from build123d import *

# Parameters (mm, degrees)
SKETCH1_R           = 4.5
BOSS_EXTRUDE1_DEPTH = 6
SKETCH3_R           = 1.6
SKETCH3_R_2         = 0.7
BOSS_EXTRUDE2_DEPTH = 1.6
SKETCH4_R           = 0.8
BOSS_EXTRUDE3_DEPTH = 0.8
BOSS_EXTRUDE4_START = -4
SKETCH5_R           = 0.6
BOSS_EXTRUDE4_DEPTH = 3
CUT_EXTRUDE1_START  = -2
CUT_EXTRUDE1_DEPTH  = 1
CUT_EXTRUDE2_START  = -4
CUT_EXTRUDE2_DEPTH  = 1
FILLET1_R           = 0.3
SKETCH6_R           = 3.2
SKETCH6_R_2         = 2.2
CUT_EXTRUDE4_DEPTH  = 2
SKETCH6_4_R         = 2.2
CUT_EXTRUDE5_DEPTH  = 19.08212732


with BuildPart() as part:
    # Sketch1 → Boss-Extrude1 (new body)
    with BuildSketch(Plane(origin=(0, 0, 0), x_dir=(1, 0, 0), z_dir=(0, 1, 0))):
        with Locations(Location((0, 0, 0), (0, 0, 270))):
            Circle(SKETCH1_R)
    extrude(amount=BOSS_EXTRUDE1_DEPTH)

    # Sketch3 → Boss-Extrude2 (add)
    # profile 1 of 4: a face of its own
    with BuildSketch(Plane.XZ):
        with Locations((-3.25, 5.629165125)):
            Circle(SKETCH3_R)
        with Locations(Location((-3.25, 5.629165125, 0), (0, 0, 270))):
            Circle(SKETCH3_R_2, mode=Mode.SUBTRACT)
    # profile 2 of 4: a face of its own
    with BuildSketch(Plane.XZ):
        with BuildLine():
            ThreePointArc((-1.65, 5.629165125), (-2.835889528, 4.083683803), (-4.635640646, 4.829165125))
            Line((-4.635640646, 4.829165125), (-3.488614731, 2.842457961))
            ThreePointArc((-3.488614731, 2.842457961), (-2.25, 3.897114317), (-0.717333438, 4.442457961))
            Line((-0.717333438, 4.442457961), (-1.864359354, 6.429165125))
            ThreePointArc((-1.864359354, 6.429165125), (-1.704518678, 6.043275597), (-1.65, 5.629165125))
        make_face()
    # profile 3 of 4: a face of its own
    with BuildSketch(Plane.XZ):
        with Locations((-3.25, -5.629165125)):
            Circle(SKETCH3_R)
        with Locations(Location((-3.25, -5.629165125, 0), (0, 0, 270))):
            Circle(SKETCH3_R_2, mode=Mode.SUBTRACT)
    # profile 4 of 4: a face of its own
    with BuildSketch(Plane.XZ):
        with BuildLine():
            ThreePointArc((-0.717333438, -4.442457961), (-2.25, -3.897114317), (-3.488614731, -2.842457961))
            Line((-3.488614731, -2.842457961), (-4.635640646, -4.829165125))
            ThreePointArc((-4.635640646, -4.829165125), (-2.835889528, -4.083683803), (-1.65, -5.629165125))
            ThreePointArc((-1.65, -5.629165125), (-1.704518678, -6.043275597), (-1.864359354, -6.429165125))
            Line((-1.864359354, -6.429165125), (-0.717333438, -4.442457961))
        make_face()
    extrude(amount=-BOSS_EXTRUDE2_DEPTH)

    # Sketch4 → Boss-Extrude3 (add, symmetric)
    with BuildSketch(Plane.XY):
        with BuildLine():
            Line((-3.5, 6), (-6.5, 6))
            ThreePointArc((-6.5, 6), (-7.9, 4.6), (-6.5, 3.2))
            Line((-6.5, 3.2), (-3.5, 3.2))
            Line((-3.5, 3.2), (-3.5, 6))
        make_face()
        with Locations((-6.5, 4.6)):
            Circle(SKETCH4_R, mode=Mode.SUBTRACT)
    extrude(amount=BOSS_EXTRUDE3_DEPTH, both=True)

    # Sketch5 → Boss-Extrude4 (add)
    # profile 1 of 2: a face of its own
    with BuildSketch(Plane(origin=(0, 6, 0), x_dir=(1, 0, 0), z_dir=(0, 1, 0)).offset(BOSS_EXTRUDE4_START)):
        with BuildLine():
            Line((4.108268481, 3.656792323), (1.029929577, 4.380553055))
            ThreePointArc((1.029929577, 4.380553055), (4.5, 0), (1.029929577, -4.380553055))
            Line((1.029929577, -4.380553055), (14.486091549, -1.216820293))
            ThreePointArc((14.486091549, -1.216820293), (15.45, 0), (14.486091549, 1.216820293))
            Line((14.486091549, 1.216820293), (12.664921694, 1.645002916))
            ThreePointArc((12.664921694, 1.645002916), (12.319323987, 1.235134702), (12.080503997, 0.75514018))
            ThreePointArc((12.080503997, 0.75514018), (11.95, 0), (12.080503997, -0.75514018))
            Line((12.080503997, -0.75514018), (4.931081365, -2.436069903))
            ThreePointArc((4.931081365, -2.436069903), (5.5, 0), (4.931081365, 2.436069903))
            ThreePointArc((4.931081365, 2.436069903), (4.560701943, 3.074084869), (4.108268481, 3.656792323))
        make_face()
        with Locations(Location((14.2, 0, 0), (0, 0, 270))):
            Circle(SKETCH5_R, mode=Mode.SUBTRACT)
    # profile 2 of 2: a face of its own
    with BuildSketch(Plane(origin=(0, 6, 0), x_dir=(1, 0, 0), z_dir=(0, 1, 0)).offset(BOSS_EXTRUDE4_START)):
        with BuildLine():
            Line((12.664921694, 1.645002916), (4.108268481, 3.656792323))
            ThreePointArc((4.108268481, 3.656792323), (4.560701943, 3.074084869), (4.931081365, 2.436069903))
            Line((4.931081365, 2.436069903), (12.080503997, 0.75514018))
            ThreePointArc((12.080503997, 0.75514018), (12.319323987, 1.235134702), (12.664921694, 1.645002916))
        make_face()
    extrude(amount=BOSS_EXTRUDE4_DEPTH)

    # Sketch5_3 → Cut-Extrude1 (cut)
    with BuildSketch(Plane(origin=(0, 6, 0), x_dir=(1, 0, 0), z_dir=(0, 1, 0)).offset(CUT_EXTRUDE1_START)):
        with BuildLine():
            Line((12.664921694, 1.645002916), (4.108268481, 3.656792323))
            ThreePointArc((4.108268481, 3.656792323), (4.560701943, 3.074084869), (4.931081365, 2.436069903))
            Line((4.931081365, 2.436069903), (12.080503997, 0.75514018))
            ThreePointArc((12.080503997, 0.75514018), (12.319323987, 1.235134702), (12.664921694, 1.645002916))
        make_face()
    extrude(amount=CUT_EXTRUDE1_DEPTH, mode=Mode.SUBTRACT)

    # Sketch5_4 → Cut-Extrude2 (cut)
    with BuildSketch(Plane(origin=(0, 6, 0), x_dir=(1, 0, 0), z_dir=(0, 1, 0)).offset(CUT_EXTRUDE2_START)):
        with BuildLine():
            Line((12.664921694, 1.645002916), (4.108268481, 3.656792323))
            ThreePointArc((4.108268481, 3.656792323), (4.560701943, 3.074084869), (4.931081365, 2.436069903))
            Line((4.931081365, 2.436069903), (12.080503997, 0.75514018))
            ThreePointArc((12.080503997, 0.75514018), (12.319323987, 1.235134702), (12.664921694, 1.645002916))
        make_face()
    extrude(amount=CUT_EXTRUDE2_DEPTH, mode=Mode.SUBTRACT)

    # Fillet1
    fillet1_edges = [part.edges().sort_by_distance(p)[0] for p in [
        (4.931081365, 3.5, 2.436069903),
        (12.080503997, 3.5, 0.75514018),
        (4.931081365, 3.5, -2.436069903),
        (12.080503997, 3.5, -0.75514018),
    ]]
    fillet(fillet1_edges, radius=FILLET1_R)

    # Sketch6 → Cut-Extrude4 (cut)
    with BuildSketch(Plane(origin=(0, 6, 0), x_dir=(1, 0, 0), z_dir=(0, 1, 0))):
        with Locations(Location((0, 0, 0), (0, 0, 270))):
            Circle(SKETCH6_R)
        with Locations(Location((0, 0, 0), (0, 0, 270))):
            Circle(SKETCH6_R_2, mode=Mode.SUBTRACT)
    extrude(amount=-CUT_EXTRUDE4_DEPTH, mode=Mode.SUBTRACT)

    # Sketch6_4 → Cut-Extrude5 (cut, through all)
    with BuildSketch(Plane(origin=(0, 6, 0), x_dir=(1, 0, 0), z_dir=(0, 1, 0))):
        with Locations(Location((0, 0, 0), (0, 0, 270))):
            Circle(SKETCH6_4_R)
    extrude(amount=-CUT_EXTRUDE5_DEPTH, mode=Mode.SUBTRACT)


solid = part.part
Source: CAD feature listing. Evaluate the final solid. Frame: model axes, mm. A direction names the side the tool comes from. Round coordinates to 2 decimals unless told otherwise and drop trailing zeros. Order: outer loops, then holes, each group sorted by start corner. A loop starts at its lowest first (then second) coordinate and runs counter-clockwise, first axis right, second up. Notation, with made-up numbers: (-10.5, 31.5) - (36.5, 31.5) arc R9 ccw to (36.5, 47.5) - close; hole circle Ø11 at (89.5, 44.25). An arc over 180 degrees is marked (long way). Use a Markdown table: item, result. Add a question column.
1. Section query B-B (z = 5.75). Return the cut outline in (x, y), then the cut area to 3 significant figures.
2. Set-up query: faces 1 (the flat face through (-4.07, 0.79, 3.85)), 2 (the flat face through (8, 4, -2)), 3 (the flat face through (-2, 1.6, -5)), 4 (the flat face through (8, 3, -2)), 5 (the cylindrical face through (-4.39, 2.96, -0.98)). Return all of +Z, -Z, +X, -X, +Y, -Y with unobstructed straight access to the full face (end or side cutting, diameter ignored); none if empty.
3. First-contact query: pin 1 (2 mm diameter, centred on x = -3, z = 4, fed in from +Y); pin 2 (3.5 mm diameter, centred on x = 7, z = -1.5, fed in from -Y); pin 3 (6 mm diameter, centred on x = 0, z = 0, fed in from +Y); pin 4 (2.5 mm diameter, centred on x = 11.5, z = -1, fed in from +Y). Flat tips, straight axial feed; report the tip coordinate or a pass-through.
4. Section query D-D (z = 1.5). Return the cut outline in (x, y).
5. Line query: probe 1 along X at (y, z) = (3.1, 0); probe 2 along X at (y, z) = (5.05, 0); probe 3 along X at (y, z) = (1.4, -5.25). Output: solid intervals per line, ascending.
6. Section query C-C (y = 4.6). Give the number of separate pieces and of enclosed holes in the cut face, then the cut area to 3 significant figures.
7. Section query A-A (x = 0). Return the cut outline in (y, z).
8. Mould query, pull axis Z, two halves, no side actions, for faces 6 (the flat face through (-1.28, 0.79, 5.42)), 7 (the flat face through (9, 5, 2)), 8 (the cylindrical face through (13.67, 3.48, 0.28)). Classes: +Z half, -Z half, draft (parallel to the pull), parting line (faces both ways), or undercut.
Derived:
| question | item | result |
|---|---|---|
| 1 | outline | (-4.85, 0) - (-3.94, 0) - (-3.94, 1.6) - (-4.85, 1.6) - close; (-2.56, 0) - (-1.47, 0) - (-1.47, 1.6) - (-2.56, 1.6) - close |
| 1 | area | 3.19 mm2 |
| 2 | face 1 | -X, +Y, -Y |
| 2 | face 2 | -Z, +Y |
| 2 | face 3 | -Z, -X, +Y |
| 2 | face 4 | -Z, -Y |
| 2 | face 5 | none |
| 3 | pin 1 | y = 6 |
| 3 | pin 2 | y = 2 |
| 3 | pin 3 | y = 4 |
| 3 | pin 4 | y = 5 |
| 4 | outline | (-4.24, 0) - (-1.61, 0) - (-1.61, 4) - (-2.83, 4) - (-2.83, 6) - (-4.24, 6) - close; (1.61, 0) - (4.24, 0) - (4.24, 2) - (5.29, 2) - (5.29, 5) - (4.24, 5) - (4.24, 6) - (2.83, 6) - (2.83, 4) - (1.61, 4) - close; (8.91, 2) - (13.28, 2) - (13.28, 5) - (8.91, 5) - close |
| 5 | probe 1 | -4.5 to -2.2, 2.2 to 5.5, 11.95 to 13.6, 14.8 to 15.45 |
| 5 | probe 2 | -7.83 to -7.16, -5.84 to -3.2, 3.2 to 4.5 |
| 5 | probe 3 | -4.8 to -3.84, -2.66 to -1.18 |
| 6 | separate pieces | 2 |
| 6 | enclosed holes | 2 |
| 6 | area | 59.0 mm2 |
| 7 | outline | (0, -4.5) - (6, -4.5) - (6, -3.2) - (4, -3.2) - (4, -2.2) - (0, -2.2) - close; (0, 2.2) - (4, 2.2) - (4, 3.2) - (6, 3.2) - (6, 4.5) - (0, 4.5) - close |
| 8 | face 6 | +Z half |
| 8 | face 7 | draft |
| 8 | face 8 | undercut |
